Source: CAD feature listing. Evaluate the final solid. Frame: model axes, mm. A direction names the side the tool comes from. Give positions to 0.01 mm unless a question says otherwise; leave off trailing zeros. Loops run counter-clockwise (first coordinate to the right, second up) from the corner with the lowest first, then second, coordinate; pieces in that order, holes last. Notation, with made-up numbers: M -34.75,-19 L -3.75,-19 A26 ccw -3.75,12 Z; hole C 9.25,62 d11. An arc over 180 degrees is marked long. Answer in a Markdown table with one row per item.
```python
from build123d import *

# Parameters (mm, degrees)
BOSS_EXTRUDE1_DEPTH = 5
BOSS_EXTRUDE2_DEPTH = 18
CUT_EXTRUDE1_DEPTH  = 1


with BuildPart() as part:
    # Sketch1 → Boss-Extrude1 (new body)
    with BuildSketch(Plane(origin=(0, 0, 0), x_dir=(1, 0, 0), z_dir=(0, 1, 0))):
        Polygon((-48.299782142, -83.657676664), (48.299782142, -83.657676664), (96.599564284, 0), (48.299782142, 83.657676664), (-48.299782142, 83.657676664), (-96.599564284, 0), align=None)
        Polygon((33.866025412, 58.657676664), (-33.866025412, 58.657676664), (-67.732050824, 0), (-33.866025412, -58.657676664), (33.866025412, -58.657676664), (67.732050824, 0), align=None, mode=Mode.SUBTRACT)
    extrude(amount=BOSS_EXTRUDE1_DEPTH)

    # Sketch1_3 → Boss-Extrude2 (add)
    with BuildSketch(Plane(origin=(0, 0, 0), x_dir=(1, 0, 0), z_dir=(0, 1, 0))):
        Polygon((-48.299782142, 83.657676664), (-96.599564284, 0), (-48.299782142, -83.657676664), (48.299782142, -83.657676664), (96.599564284, 0), (48.299782142, 83.657676664), align=None)
        Polygon((-85.0525589, 0), (-42.52627945, -73.657676664), (42.52627945, -73.657676664), (85.0525589, 0), (42.52627945, 73.657676664), (-42.52627945, 73.657676664), align=None, mode=Mode.SUBTRACT)
    extrude(amount=BOSS_EXTRUDE2_DEPTH)

    # Sketch2 → Cut-Extrude1 (cut)
    with BuildSketch(Plane(origin=(0, 14.35, 0), x_dir=(1, 0, 0), z_dir=(0, 1, 0))):
        Polygon((86.207259438, 0), (43.103629719, 74.657676664), (-43.103629719, 74.657676664), (-86.207259438, 0), (-43.103629719, -74.657676664), (43.103629719, -74.657676664), align=None)
        Polygon((85.0525589, 0), (42.52627945, 73.657676664), (-42.52627945, 73.657676664), (-85.0525589, 0), (-42.52627945, -73.657676664), (42.52627945, -73.657676664), align=None, mode=Mode.SUBTRACT)
    extrude(amount=CUT_EXTRUDE1_DEPTH, mode=Mode.SUBTRACT)


solid = part.part
```
Q1. Section query C-C (z = -9). Output: boundary loops of the cut face in (x, y).
Values follow:
| item | result |
|---|---|
| outline | M -91.4,0 L -62.54,0 L -62.54,5 L -79.86,5 L -79.86,14.35 L -81.01,14.35 L -81.01,15.35 L -79.86,15.35 L -79.86,18 L -91.4,18 Z; M 62.54,0 L 91.4,0 L 91.4,18 L 79.86,18 L 79.86,15.35 L 81.01,15.35 L 81.01,14.35 L 79.86,14.35 L 79.86,5 L 62.54,5 Z |
Q2. Contact query for flat-ended pins moving along their axis: pin 1 Ø5 at (x, y) = (66.5, 14.5) entering from -Z; pin 2 Ø10 at (x, y) = (-71, 2) entering from -Z; pin 3 Ø10 at (y, z) = (4.5, 44) entering from -X. Output: stop coordinate, or through.
Values follow:
| item | result |
|---|---|
| pin 1 | z = -56.46 |
| pin 2 | z = -53 |
| pin 3 | x = -74.08 |
Q3. Section query B-B (y = 8.5). Output: boundary loops of the cut face in (x, z).
Values follow:
| item | result |
|---|---|
| outline | M -96.6,0 L -48.3,-83.66 L 48.3,-83.66 L 96.6,0 L 48.3,83.66 L -48.3,83.66 Z; hole M -85.05,0 L -42.53,-73.66 L 42.53,-73.66 L 85.05,0 L 42.53,73.66 L -42.53,73.66 Z |
Q4. Ray query, probe 1 along Z at (x, y) = (26, 7.75); probe 2 along Z at (x, y) = (28, 4.25); probe 3 along Y at (x, z) = (53, -34). Return the intervals inside material, ascending. Write a range as from..to.
Values follow:
| item | result |
|---|---|
| probe 1 | -83.66..-73.66, 73.66..83.66 |
| probe 2 | -83.66..-58.66, 58.66..83.66 |
| probe 3 | 0..5 |
Q5. Section query D-D (x = -75). Output: boundary loops of the cut face in (y, z), plus the area to 3 significant figures.
Values follow:
| item | result |
|---|---|
| outline | M 0,-37.41 L 18,-37.41 L 18,-17.41 L 15.35,-17.41 L 15.35,-19.41 L 14.35,-19.41 L 14.35,-17.41 L 5,-17.41 L 5,17.41 L 14.35,17.41 L 14.35,19.41 L 15.35,19.41 L 15.35,17.41 L 18,17.41 L 18,37.41 L 0,37.41 Z |
| area | 890 mm^2 |
Q6. Mould query, pull axis X, two halves, no side actions, for faces 1 (the flat face through (64.09, 16.66, -36.31)), 2 (the flat face through (-1, 9, 83.658)), 3 (the flat face through (72.112, 8.874, 42.414)). Classes: +X half, -X half, draft (parallel to the pull), parting line (faces both ways), or undercut.
Values follow:
| item | result |
|---|---|
| face 1 | undercut |
| face 2 | draft |
| face 3 | +X half |
Q7. Reachability of faces 4 (the flat face through (64.957, 14.843, -36.806)), 5 (the flat face through (63.492, 16.656, 37.344)), 6 (the flat face through (51.036, 2.465, -28.918)) from +Z, -Z, +X, -X, +Y, -Y: full face, straight path, thin tool, end or side. Return the list, or none.
Values follow:
| item | result |
|---|---|
| face 4 | none |
| face 5 | +Y |
| face 6 | +Y, -Y |
Q8. Section query A-A (x = 8). Output: boundary loops of the cut face in (y, z), plus the area to 3 significant figures.
Values follow:
| item | result |
|---|---|
| outline | M 0,-83.66 L 18,-83.66 L 18,-73.66 L 15.35,-73.66 L 15.35,-74.66 L 14.35,-74.66 L 14.35,-73.66 L 5,-73.66 L 5,-58.66 L 0,-58.66 Z; M 0,58.66 L 5,58.66 L 5,73.66 L 14.35,73.66 L 14.35,74.66 L 15.35,74.66 L 15.35,73.66 L 18,73.66 L 18,83.66 L 0,83.66 Z |
| area | 508 mm^2 |
